Geometry: see drawing. Coordinates: mm, zero at the bounding-box minimum. A direction names the side the tool comes from. Coordinates: 2 decimals unless noted, no trailing zeros. Write each loop counter-clockwise with the first axis right and the second up, starting at its lowest first coordinate (ties: lowest second). Pieces come first, ordered by that corner, then holes. Notation, with made-up numbers: (36.5, 73) -> (66.5, 73) arc R19 cw to (66.5, 101) -> close; hole circle Ø9 at (54.5, 25). An arc over 180 degrees is marked (long way). Use one line per item in the form item = value. Start each with the question number.
(1) Cut plane D-D on y = 25. Return the cut outline in (x, z).
(2) First-contact query: pin 1 (1.1 mm diameter, centred on x = 0.5, z = 9.5, fed in from +Y); pin 2 (1.5 mm diameter, centred on x = 14, y = 17.5, fed in from -Z); pin 3 (0.8 mm diameter, centred on x = 0.5, z = 11, fed in from -Y). Flat tips, straight axial feed; report the tip coordinate or a pass-through.
(3) Ray query, line 1 along X through (y, z) = (30.5, 4); line 2 along Y through (x, z) = (9.5, 8.25); line 3 along X through (y, z) = (23, 4.25). Return the intervals inside material, ascending.
(4) Cut plane A-A on x = 5. Return the cut outline in (y, z), plus the area to 3 significant figures.
(5) Set-up query: the marked faces 1 and 2. Return all of +Z, -Z, +X, -X, +Y, -Y with unobstructed straight access to the full face (end or side cutting, diameter ignored); none if empty.
(6) Cut plane C-C on z = 2. Return the cut outline in (x, y).
(7) Cut plane B-B on y = 30.5. Return the cut outline in (x, z).
(8) Pull-direction query (Y, two-part tool) for the marked faces 3, 4 and 5; classes: released by +Y, released by -Y, zero draft, split by the parting line, or undercut.
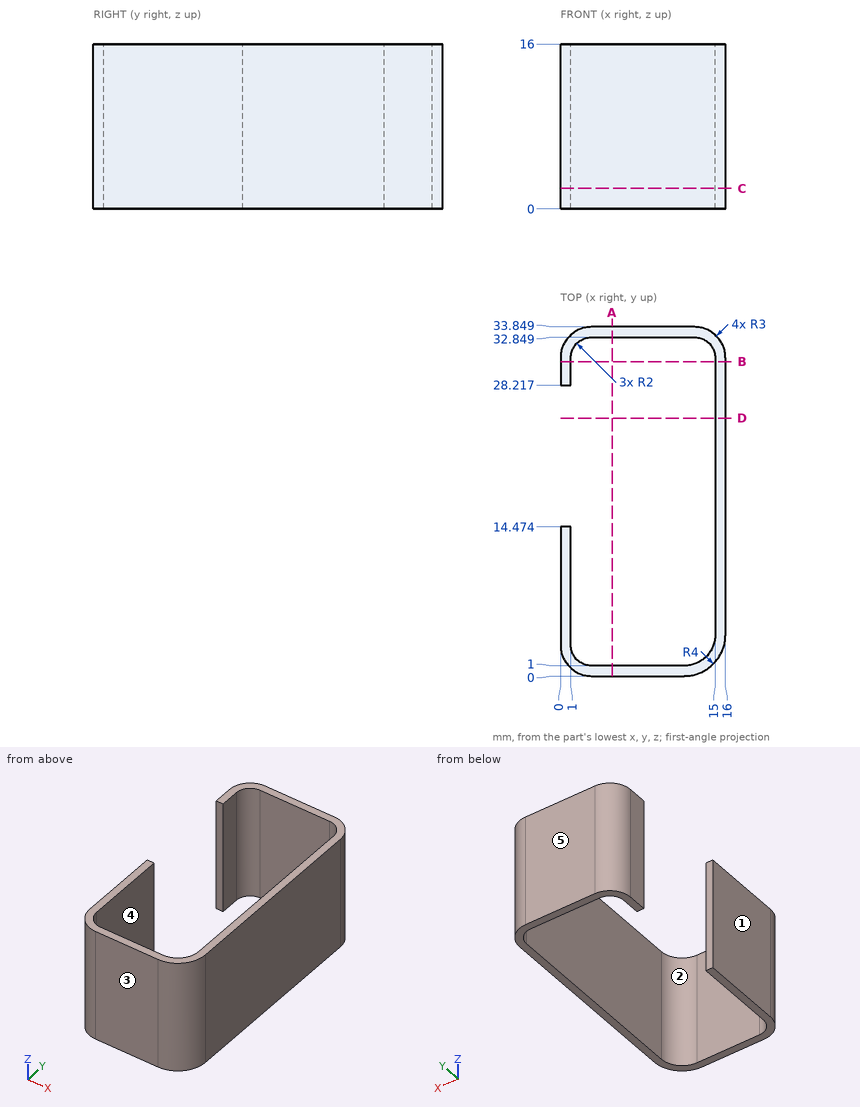
Values:
q1.outline = (15, 0) -> (16, 0) -> (16, 16) -> (15, 16) -> close
q2.pin_1 = 33.13
q2.pin_2 = through
q2.pin_3 = 0.86
q3.line_1 = 0 to 1, 15 to 16
q3.line_2 = 0 to 1, 32.85 to 33.85
q3.line_3 = 15 to 16
q4.outline = (0, 0) -> (1, 0) -> (1, 16) -> (0, 16) -> close; (32.85, 0) -> (33.85, 0) -> (33.85, 16) -> (32.85, 16) -> close
q4.area = 32.0 mm2
q5.face_1 = +Z, -Z, -X, +Y, -Y
q5.face_2 = +Z, -Z
q6.outline = (0, 3) arc R3 ccw to (3, 0) -> (12, 0) arc R4 ccw to (16, 4) -> (16, 30.85) arc R3 ccw to (13, 33.85) -> (3, 33.85) arc R3 ccw to (0, 30.85) -> (0, 28.22) -> (1, 28.22) -> (1, 30.85) arc R2 cw to (3, 32.85) -> (13, 32.85) arc R2 cw to (15, 30.85) -> (15, 4) arc R3 cw to (12, 1) -> (3, 1) arc R2 cw to (1, 3) -> (1, 14.47) -> (0, 14.47) -> close
q7.outline = (0, 0) -> (1, 0) -> (1, 16) -> (0, 16) -> close; (15, 0) -> (16, 0) -> (16, 16) -> (15, 16) -> close
q8.face_3 = released by -Y
q8.face_4 = undercut
q8.face_5 = released by +Y
